from build123d import *

# Parameters (mm, degrees)
SKETCH1_R           = 5
BOSS_EXTRUDE1_DEPTH = 5


with BuildPart() as part:
    # Sketch1 → Boss-Extrude1 (new body, symmetric)
    with BuildSketch(Plane(origin=(0, 0, 0), x_dir=(0, 0, -1), z_dir=(1, 0, 0))):
        with BuildLine():
            Line((0, 15), (30, 15))
            Line((30, 15), (30, -15))
            Line((30, -15), (0, -15))
            ThreePointArc((0, -15), (-15, 0), (0, 15))
        make_face()
        Circle(SKETCH1_R, mode=Mode.SUBTRACT)
    extrude(amount=BOSS_EXTRUDE1_DEPTH, both=True)

    # Sketch3 → Revolve1 (revolve)
    with BuildSketch(Plane(origin=(5, 0, 0), x_dir=(0, 0, -1), z_dir=(1, 0, 0))):
        Polygon((30, 15), (30, 20.753758682), (33.999504278, 20.753758682), (33.999504278, 15), (283.999504278, 15), (283.999504278, 0), (30, 0), align=None)
    revolve(axis=Axis((5, 0, -283.999504278), (0, 0, 1)))


solid = part.part
Here's how the part is built. I have some questions about the finished solid (model axes, mm). A direction names the side the tool comes from. Coordinates: 2 decimals unless noted, no trailing zeros. Order: outer loops, then holes, each group sorted by start corner. A loop starts at its lowest first (then second) coordinate and runs counter-clockwise, first axis right, second up. Notation, with made-up numbers: M 70.25,38 L 100.25,38 A17 ccw 100.25,56 Z; hole C 37,44.5 d3. An arc over 180 degrees is marked long. Answer as CSV lines item,"result".
Item 1: Imagine slicing it at A-A on y = 0. Write out the boundary of the cut face in (x, z), plus the area to 3 significant figures.
Results found:
outline,"M -15.75,-34 L -10,-34 L -10,-284 L 20,-284 L 20,-34 L 25.75,-34 L 25.75,-30 L 5,-30 L 5,-5 L -5,-5 L -5,-30 L -15.75,-30 Z; M -5,5 L 5,5 L 5,15 L -5,15 Z"
area,"8,020 mm2"
Item 2: On a 3-axis mill with a long thin cutter (end or side, diameter ignored), from which of +Z, -Z, +X, -X, +Y, -Y can I reach the whole of each face in a straight line? I mean faces 4 (the face through (-5, 0, -8)), 5 (the face through (0, -15, -15)), 6 (the face through (0, 15, -15)), 7 (the face through (4.34, -14.985, -160.75)). Say none if no direction works.
Results found:
face 4,"+Z, -X, +Y, -Y"
face 5,"+Z, +X, -X, -Y"
face 6,"+Z, +X, -X, +Y"
face 7,"-Z"
Item 3: Imagine slicing it at D-D on z = -95.5. Write out the boundary of the cut face in (x, y), plus the area to 3 significant figures.
Results found:
outline,"C 5,0 d30"
area,"707 mm2"
Item 4: We'd pull the mould along Z, two halves only. Please class faces 1 (the face through (0, 0, 15)), 2 (the face through (-0.07, -4.88, 1.08)), 3 (the face through (5, 0, -8)): +Z half, -Z half, draft (parallel to the pull), parting line (faces both ways), or undercut.
Results found:
face 1,"+Z half"
face 2,"undercut"
face 3,"draft"
Item 5: If I drill on line 1 (Z direction, x = -12, y = -6); line 2 (Z direction, x = 16.5, y = -3.5); line 3 (X direction, y = 1, z = -111), over which ranges is the centre line in solid material (lowest first)?
Results found:
line 1,"-34 to -30"
line 2,"-284 to -30"
line 3,"-9.97 to 19.97"
Item 6: For pin 1 (1 mm diameter, centred on y = 7.5, z = -33, fed in from -X); pin 2 (24 mm diameter, centred on y = -3, z = -5, fed in from +X); pin 3 (1.5 mm diameter, centred on x = 18, z = -120, fed in from -Y); pin 4 (8 mm diameter, centred on y = 0, z = 0, fed in from -X), each with a flat end and sliding along its axis, tell me the tip position at first contact or that it passes through.
Results found:
pin 1,"x = -14.54"
pin 2,"x = 5"
pin 3,"y = -8.66"
pin 4,"through"
Item 7: Imagine slicing it at B-B on x = 0.5. Write out the boundary of the cut face in (y, z), plus the area to 3 significant figures.
Results found:
outline,"M -20.26,-34 L -14.31,-34 L -14.31,-284 L 14.31,-284 L 14.31,-34 L 20.26,-34 L 20.26,-30 L 15,-30 L 15,0 A15 ccw -15,0 L -15,-30 L -20.26,-30 Z; hole C 0,0 d10"
area,"8,490 mm2"
Item 8: Imagine slicing it at C-C on y = 11. Write out the boundary of the cut face in (x, z), plus the area to 3 significant figures.
Results found:
outline,"M -12.6,-34 L -5.2,-34 L -5.2,-284 L 15.2,-284 L 15.2,-34 L 22.6,-34 L 22.6,-30 L 5,-30 L 5,10.2 L -5,10.2 L -5,-30 L -12.6,-30 Z"
area,"5,640 mm2"
